The listing builds one solid part. Answer for the finished solid, in the listing's coordinates (mm). Face numbers are marked on the shaded views. A direction names the side the tool comes from. Coordinates: 2 decimals unless noted, no trailing zeros. Order: outer loops, then holes, each group sorted by start corner. A loop starts at its lowest first (then second) coordinate and runs counter-clockwise, first axis right, second up.
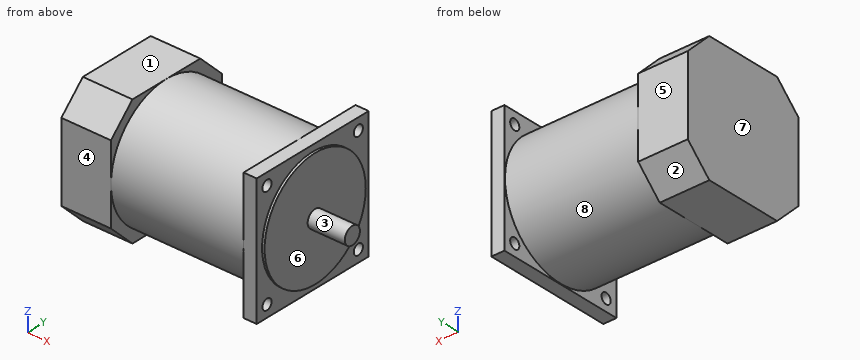
from build123d import *

# Parameters (mm, degrees)
F0_W      = 104
F0_H      = 104
F1_DEPTH  = 160
F3_W      = 107.42
F3_H      = 40
F5_W      = 104
F5_H      = 104
F5_W_2    = 103
F5_H_2    = 103
F6_DEPTH  = 40
F7_SIZE   = 20
F8_R      = 4.25
F9_DEPTH  = 25
F10_R     = 7
F11_DEPTH = 30
F12_W     = 104
F12_H     = 104
F12_R     = 4.25
F12_R_2   = 47
F13_DEPTH = 2


with BuildPart() as f1:
    # F0 (on Right) → F1 (new body)
    with BuildSketch(Plane.YZ):
        with Locations((52, 52)):
            Rectangle(F0_W, F0_H)
    extrude(amount=-F1_DEPTH)

    # F3 (on offset) → F4 (revolve, cut)
    with BuildSketch(Plane.XZ.offset(-52)):
        with Locations((-66.29, 123.5)):
            Rectangle(F3_W, F3_H)
    revolve(axis=Axis((-69.2846309394, 52, 52), (1, 0, 0)), mode=Mode.SUBTRACT)

    # F5 (on face) → F6 (cut)
    with BuildSketch(Plane(origin=(-160, 0, 0), x_dir=(0, -1, 0), z_dir=(-1, 0, 0))):
        with Locations((-52, 52)):
            Rectangle(F5_W, F5_H)
        with Locations((-52, 52)):
            Rectangle(F5_W_2, F5_H_2, mode=Mode.SUBTRACT)
    extrude(amount=-F6_DEPTH, mode=Mode.SUBTRACT)

    # F7
    f7_edges = [f1.edges().sort_by_distance(p)[0] for p in [
        (-140, 0.5, 103.5),
        (-140, 103.5, 103.5),
        (-140, 103.5, 0.5),
        (-140, 0.5, 0.5),
    ]]
    chamfer(f7_edges, length=F7_SIZE)

    # F8 (on face) → F9 (cut)
    with BuildSketch(Plane.YZ):
        with Locations((94.4264068712, 94.4264068712)):
            Circle(F8_R)
        with Locations((94.4264068712, 9.5735931288)):
            Circle(F8_R)
        with Locations((9.5735931288, 94.4264068712)):
            Circle(F8_R)
        with Locations((9.5735931288, 9.5735931288)):
            Circle(F8_R)
    extrude(amount=-F9_DEPTH, mode=Mode.SUBTRACT)

    # F10 (on face) → F11 (join)
    with BuildSketch(Plane.YZ):
        with Locations((52, 52)):
            Circle(F10_R)
    extrude(amount=F11_DEPTH)

    # F12 (on face) → F13 (cut)
    with BuildSketch(Plane.YZ):
        with Locations((52, 52)):
            Rectangle(F12_W, F12_H)
        with Locations((9.5735931288, 9.5735931288)):
            Circle(F12_R, mode=Mode.SUBTRACT)
        with Locations((94.4264068712, 9.5735931288)):
            Circle(F12_R, mode=Mode.SUBTRACT)
        with Locations((9.5735931288, 94.4264068712)):
            Circle(F12_R, mode=Mode.SUBTRACT)
        with Locations((52, 52)):
            Circle(F12_R_2, mode=Mode.SUBTRACT)
        with Locations((94.4264068712, 94.4264068712)):
            Circle(F12_R, mode=Mode.SUBTRACT)
    extrude(amount=-F13_DEPTH, mode=Mode.SUBTRACT)


solid = f1.part
1) Determine the mould class of the marked faces 5, 6, 7 and 8 for opening direction X: released by +X, released by -X, zero draft, split by the parting line, or undercut.
2) Section B-B (z = 76.5) is taken. Give the vertices of the cut face in (x, y).
3) Each of these flat-tipped pins is pushed along its axis until it touches: P1, Ø12, axis at x = -107.5, z = 15.5, coming from the -Y side; P2, Ø6, axis at x = -62, z = 81.5, coming from the +Y side; P3, Ø12, axis at x = -139, z = 44, coming from the -Y side. Where does it stop, or does it pass through?
4) Section C-C (x = -100) is taken. Give the vertices of the cut face in (y, z).
5) Consider L1, parallel to Y at x = -6, z = 9; L2, parallel to X at y = 11.5, z = 86.5; L3, parallel to X at y = 66, z = 62. Determine where each line is inside the solid, lowest interval first.
6) A tool of negligible diameter and unlimited length cuts with its end or side. For the marked faces 1, 2, 3 and 4, from which of +Z, -Z, +X, -X, +Y, -Y can it reach the whole face along a straight path? Write none if from no direction.
7) Section D-D (z = 47) is taken. Give the vertices of the cut face in (x, y).
8) Section A-A (y = 65) is taken. Give the vertices of the cut face in (x, z).
Filled sheet:
1. face 5: zero draft
1. face 6: released by +X
1. face 7: released by -X
1. face 8: undercut
2. outline: (-160, 0.5) - (-120, 0.5) - (-120, 6.7) - (-12.58, 6.7) - (-12.58, 0) - (-2, 0) - (-2, 11.89) - (0, 11.89) - (0, 92.11) - (-2, 92.11) - (-2, 104) - (-12.58, 104) - (-12.58, 97.3) - (-120, 97.3) - (-120, 103.5) - (-160, 103.5) - close
3. P1: stops at y = 10.5
3. P2: stops at y = 96.16
3. P3: stops at y = 0.5
4. outline: circle Ø103 at (52, 52)
5. L1: y = 0 to 5.36, 13.78 to 90.22, 98.64 to 104
5. L2: x = -160 to -120, -12.58 to -2
5. L3: x = -160 to 0
6. face 1: +Z, -X, +Y, -Y
6. face 2: -Z, -X, +Y
6. face 3: +X
6. face 4: +Z, -Z, -X, -Y
7. outline: (-160, 0.5) - (-120, 0.5) - (-120, 0.74) - (-12.58, 0.74) - (-12.58, 0) - (-2, 0) - (-2, 5.27) - (0, 5.27) - (0, 47.1) - (30, 47.1) - (30, 56.9) - (0, 56.9) - (0, 98.73) - (-2, 98.73) - (-2, 104) - (-12.58, 104) - (-12.58, 103.26) - (-120, 103.26) - (-120, 103.5) - (-160, 103.5) - close
8. outline: (-160, 0.5) - (-120, 0.5) - (-120, 2.17) - (-12.58, 2.17) - (-12.58, 0) - (-2, 0) - (-2, 6.83) - (0, 6.83) - (0, 97.17) - (-2, 97.17) - (-2, 104) - (-12.58, 104) - (-12.58, 101.83) - (-120, 101.83) - (-120, 103.5) - (-160, 103.5) - close
